from build123d import *

# Parameters (mm, degrees)
BOSS_EXTRUDE1_DEPTH                           = 9.5
CBORE_FOR_M12_HEX_HEAD_CAP_SCREW1_D           = 6.75
CBORE_FOR_M12_HEX_HEAD_CAP_SCREW1_CBORE_D     = 25
CBORE_FOR_M12_HEX_HEAD_CAP_SCREW1_CBORE_DEPTH = 3


with BuildPart() as part:
    # Sketch2 → Boss-Extrude1 (new, symmetric)
    with BuildSketch(Plane.XY):
        with BuildLine():
            Line((12.7, 0), (25.4, 0))
            Line((25.4, 0), (25.4, 19))
            Line((25.4, 19), (-25.4, 19))
            Line((-25.4, 19), (-25.4, 0))
            Line((-25.4, 0), (-12.7, 0))
            ThreePointArc((-12.7, 0), (0, 12.7), (12.7, 0))
        make_face()
    extrude(amount=BOSS_EXTRUDE1_DEPTH, both=True)

    # CBORE for M12 Hex Head Cap Screw1 (through all)
    with Locations(Plane(origin=(0, 19, 0), x_dir=(1, 0, 0), z_dir=(0, 1, 0))):
        with Locations((-19.05, 0), (19.05, 0)):
            CounterBoreHole(CBORE_FOR_M12_HEX_HEAD_CAP_SCREW1_D / 2, CBORE_FOR_M12_HEX_HEAD_CAP_SCREW1_CBORE_D / 2, CBORE_FOR_M12_HEX_HEAD_CAP_SCREW1_CBORE_DEPTH)


solid = part.part
Design review of the part built by this model. Coordinates are the model's own, in mm. A direction names the side the tool comes from. Round coordinates to 2 decimals unless told otherwise and drop trailing zeros. Order: outer loops, then holes, each group sorted by start corner. A loop starts at its lowest first (then second) coordinate and runs counter-clockwise, first axis right, second up.
1) Clearance check with flat-ended pins moving along their axes: pin 1 Ø5.5 at (x, z) = (-17, -4) entering from +Y; pin 2 Ø6 at (x, z) = (0, 6) entering from -Y; pin 3 Ø1 at (x, z) = (0.5, 5.5) entering from -Y. State where each tip first meets the part, or that it passes through.
The answers:
pin 1: stops at y = 16
pin 2: stops at y = 12.34
pin 3: stops at y = 12.66
2) Consider section D-D (y = 14.25). State the section outline as (x, z) points (3 decimals).
The answers:
outline: (-25.4, -9.5) - (25.4, -9.5) - (25.4, 9.5) - (-25.4, 9.5) - close; hole circle Ø6.75 at (-19.05, 0); hole circle Ø6.75 at (19.05, 0)
3) Consider section B-B (x = 19.05). State the section outline as (y, z) points (3 decimals).
The answers:
outline: (0, -9.5) - (16, -9.5) - (16, -3.375) - (0, -3.375) - close; (0, 3.375) - (16, 3.375) - (16, 9.5) - (0, 9.5) - close
4) For L1, parallel to Z at x = -19.05, y = 7.5 (3 decimals); L2, parallel to X at y = 14.25, z = 1.25; L3, parallel to X at y = 4, z = -2.25, list the stretches that pass through material, from the lowest coordinate up.
The answers:
L1: z = -9.5 to -3.375, 3.375 to 9.5
L2: x = -25.4 to -22.18, -15.92 to 15.92, 22.18 to 25.4
L3: x = -25.4 to -21.57, -16.53 to -12.05, 12.05 to 16.53, 21.57 to 25.4
5) Draft analysis for pull direction X (two halves, no side actions). For faces 1 (the cylindrical face through (6.55, 17.52, -0.15)), 2 (the cylindrical face through (-6.55, 17.52, 0.15)), 3 (the flat face through (16, 0, 2)), 4 (the cylindrical face through (-15.68, 7.89, -0.15)), state which applies: released by +X, released by -X, zero draft, split by the parting line, or undercut.
The answers:
face 1: released by +X
face 2: released by -X
face 3: zero draft
face 4: undercut
6) Machinability: for faces 5 (the flat face through (-16, 16, 2)), 6 (the flat face through (0, 14, 9.5)), 7 (the flat face through (16, 16, -2)), which of the approach directions +Z, -Z, +X, -X, +Y, -Y give a long, thin tool a straight path to every point of the face, cutting with its end or side? Answer none if there is none.
The answers:
face 5: -X, +Y
face 6: +Z, +X, -X, +Y, -Y
face 7: +X, +Y
7) Consider section A-A (z = 0). State the section outline as (x, y) points (3 decimals), plus the area to 3 significant figures.
The answers:
outline: (-25.4, 0) - (-22.425, 0) - (-22.425, 16) - (-25.4, 16) - close; (-15.675, 0) - (-12.7, 0) arc R12.7 cw to (12.7, 0) - (15.675, 0) - (15.675, 16) - (6.55, 16) - (6.55, 19) - (-6.55, 19) - (-6.55, 16) - (-15.675, 16) - close; (22.425, 0) - (25.4, 0) - (25.4, 16) - (22.425, 16) - close
area: 383 mm2
8) Consider section C-C (y = 8.5). State the section outline as (x, z) points (3 decimals).
The answers:
outline: (-25.4, -9.5) - (-9.436, -9.5) - (-9.436, 9.5) - (-25.4, 9.5) - close; (9.436, -9.5) - (25.4, -9.5) - (25.4, 9.5) - (9.436, 9.5) - close; hole circle Ø6.75 at (-19.05, 0); hole circle Ø6.75 at (19.05, 0)
